Could you check a few things on this drawing? It's one solid part, dimensions in mm from its lowest x, y, z. A direction names the side the tool comes from. Round coordinates to 2 decimals unless told otherwise and drop trailing zeros. Order: outer loops, then holes, each group sorted by start corner. A loop starts at its lowest first (then second) coordinate and runs counter-clockwise, first axis right, second up. Notation, with made-up numbers: M 0.5,70 L 59.5,70 A8 ccw 59.5,83 Z; hole C -28.75,35 d7. An arc over 180 degrees is marked long. Answer as a JSON object with one key per item and string values. Group by question number.
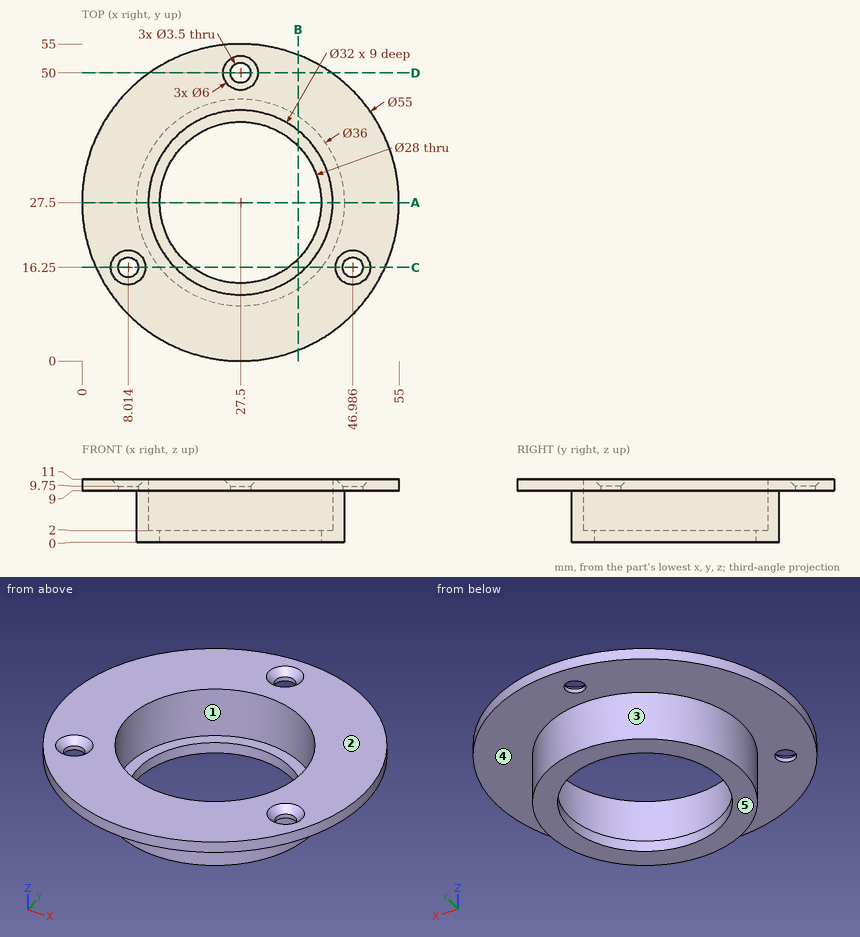
1) If we section it at D-D on y = 50: Write out the boundary of the cut face in (x, z).
2) I need wall thicknesses on line 1 along Y through (x, z) = (27.5, 9.5); line 2 along Y through (x, z) = (27.5, 4.5); line 3 along Y through (x, z) = (27.5, 0.95). Which ranges of each line are inside material? Lowest first, please.
3) Which directions (+Z, -Z, +X, -X, +Y, -Y) give clear straight access to the entire face, cutting with the end or side of a thin tool? Please do the marked faces 4 and 5.
4) If we section it at A-A on y = 27.5: Write out the boundary of the cut face in (x, z).
5) We'd pull the mould along X, two halves only. Please class the marked faces 1, 2 and 3: +X half, -X half, draft (parallel to the pull), parting line (faces both ways), or undercut.
6) For pin 1 (1 mm diameter, centred on y = 23.5, z = 2.5, fed in from -X); pin 2 (6 mm diameter, centred on y = 20.5, z = 7, fed in from +X); pin 3 (2 mm diameter, centred on x = 8.01, y = 16.25, fed in from -Z); pin 4 (4 mm diameter, centred on x = 27.5, y = 50, fed in from +Z), each with a flat end and sliding along its axis, tell me the tip position at first contact or that it passes through.
7) If we section it at B-B on x = 37.5: Write out the boundary of the cut face in (y, z), plus the area to 3 significant figures.
8) If we section it at C-C on y = 16.25: Count the separate pieces of the cut face and the enclosed holes in it.
Findings:
{
 "1": {"outline": "M 11.69,9 L 25.75,9 L 25.75,9.75 L 24.5,11 L 11.69,11 Z; M 29.25,9 L 43.31,9 L 43.31,11 L 30.5,11 L 29.25,9.75 Z"},
 "2": {"line 1": "y = 0 to 11.5, 43.5 to 48.25, 51.75 to 55", "line 2": "y = 9.5 to 11.5, 43.5 to 45.5", "line 3": "y = 9.5 to 13.5, 41.5 to 45.5"},
 "3": {"face 4": "-Z", "face 5": "-Z, +X, -X, +Y, -Y"},
 "4": {"outline": "M 0,9 L 9.5,9 L 9.5,0 L 13.5,0 L 13.5,2 L 11.5,2 L 11.5,11 L 0,11 Z; M 41.5,0 L 45.5,0 L 45.5,9 L 55,9 L 55,11 L 43.5,11 L 43.5,2 L 41.5,2 Z"},
 "5": {"face 1": "undercut", "face 2": "draft", "face 3": "parting line"},
 "6": {"pin 1": "stops at x = 9.84", "pin 2": "stops at x = 54.58", "pin 3": "passes through", "pin 4": "stops at z = 10"},
 "7": {"outline": "M 1.88,9 L 12.53,9 L 12.53,0 L 17.7,0 L 17.7,2 L 15.01,2 L 15.01,11 L 1.88,11 Z; M 37.3,0 L 42.47,0 L 42.47,9 L 53.12,9 L 53.12,11 L 39.99,11 L 39.99,2 L 37.3,2 Z", "area": "108 mm^2"},
 "8": {"separate pieces": "4", "enclosed holes": "0"}
}
